from build123d import *

# Parameters (mm, degrees)
CROQUIS1_R              = 2.75
SALIENTE_EXTRUIR1_DEPTH = 6
SALIENTE_EXTRUIR2_DEPTH = 12
CORTAR_EXTRUIR1_DEPTH   = 4


with BuildPart() as part:
    # Croquis1 → Saliente-Extruir1 (new body)
    with BuildSketch(Plane.XY):
        Polygon((-9.5, 11.2), (-14, 11.2), (-14, 0), (0, 0), (0, 11.2), (-4.5, 11.2), (-4.5, 15.2), (-9.5, 15.2), align=None)
        with Locations((-7, 6)):
            Circle(CROQUIS1_R, mode=Mode.SUBTRACT)
    extrude(amount=SALIENTE_EXTRUIR1_DEPTH)

    # Croquis2 → Saliente-Extruir2 (add)
    with BuildSketch(Plane(origin=(0, 15.2, 0), x_dir=(1, 0, 0), z_dir=(0, 1, 0))):
        with BuildLine():
            Line((-9.5, 0), (-4.5, 0))
            ThreePointArc((-4.5, 0), (-7, -2.5), (-9.5, 0))
        make_face()
    extrude(amount=SALIENTE_EXTRUIR2_DEPTH)

    # Croquis3 → Cortar-Extruir1 (cut)
    with BuildSketch(Plane.XY.offset(6)):
        Polygon((-2.092522712, 6), (-4.546261356, 10.25), (-9.453738644, 10.25), (-11.907477288, 6), (-9.453738644, 1.75), (-4.546261356, 1.75), align=None)
    extrude(amount=-CORTAR_EXTRUIR1_DEPTH, mode=Mode.SUBTRACT)


solid = part.part
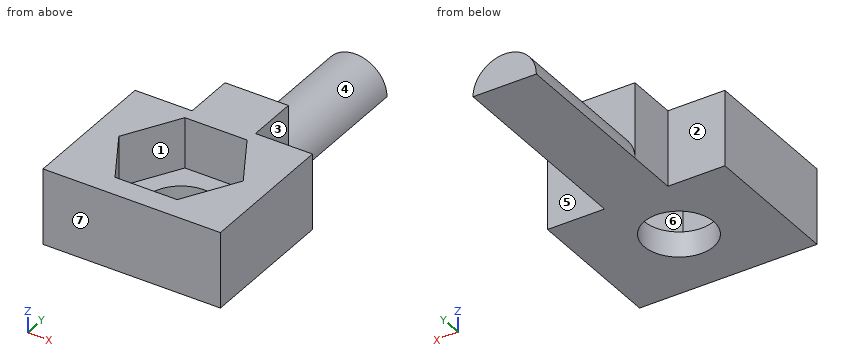
Can you work these out from the model? Positions are in its coordinate system, mm. Face numbers are marked on the shaded views. A direction names the side the tool comes from. Coordinates: 2 decimals unless noted, no trailing zeros. Write each loop counter-clockwise with the first axis right and the second up, starting at its lowest first coordinate (ties: lowest second). Pieces come first, ordered by that corner, then holes. Notation, with made-up numbers: M 44,76.5 L 58,76.5 A12 cw 58,97.5 Z; hole C 36.5,-7.75 d1. An arc over 180 degrees is marked long. Use one line per item in the form item = value.
Q1. I need wall thicknesses on line 1 along X through (y, z) = (6, 1.1); line 2 along Y through (x, z) = (-7, 1.05); line 3 along Y through (x, z) = (-4.75, 4). Which ranges of each line are inside material? Lowest first, please. Write a range as from..to.
Model answer:
line_1 = -14..-9.75, -4.25..0
line_2 = 0..3.25, 8.75..27.2
line_3 = 0..1.75, 10.25..15.2
Q2. If we section it at C-C (y = 4.5): Write out the boundary of the cut face in (x, z).
Model answer:
outline = M -14,0 L -9.3,0 L -9.3,2 L -11.04,2 L -11.04,6 L -14,6 Z; M -4.7,0 L 0,0 L 0,6 L -2.96,6 L -2.96,2 L -4.7,2 Z
Q3. For the marked faces 1, 2, 3 and 4, which set-ups out of +Z, -Z, +X, -X, +Y, -Y let a thin tool reach every point of the face, with its end or its side?
Model answer:
face_1 = +Z
face_2 = +Z, -Z, -X, +Y
face_3 = +Z, -Z, +X, +Y
face_4 = +Z, +Y
Q4. If we section it at A-A (x = -7): Write out the boundary of the cut face in (y, z), then the cut area to 3 significant figures.
Model answer:
outline = M 0,0 L 3.25,0 L 3.25,2 L 1.75,2 L 1.75,6 L 0,6 Z; M 8.75,0 L 27.2,0 L 27.2,2.5 L 15.2,2.5 L 15.2,6 L 10.25,6 L 10.25,2 L 8.75,2 Z
area = 76.2 mm^2
Q5. We'd pull the mould along Y, two halves only. Please class the marked faces 5, 6 and 7: +Y half, -Y half, draft (parallel to the pull), parting line (faces both ways), or undercut.
Model answer:
face_5 = +Y half
face_6 = undercut
face_7 = -Y half
Q6. If we section it at B-B (z = 4.85): Write out the boundary of the cut face in (x, y), then the cut area to 3 significant figures.
Model answer:
outline = M -14,0 L 0,0 L 0,11.2 L -4.5,11.2 L -4.5,15.2 L -9.5,15.2 L -9.5,11.2 L -14,11.2 Z; hole M -11.91,6 L -9.45,1.75 L -4.55,1.75 L -2.09,6 L -4.55,10.25 L -9.45,10.25 Z
area = 114 mm^2
Q7. For P1, Ø4, axis at x = -9, y = 6.5, coming from the +Z side; P2, Ø1.5, axis at x = -7, y = 6.5, coming from the -Z side; P3, Ø3.5, axis at x = -12, z = 2, coming from the +Y side; P4, Ø3, axis at x = -7.5, z = 4.5, coming from the -Y side, each with a flat end and sliding along its axis, tell me the tip position at first contact or that it passes through.
Model answer:
P1 = 2
P2 = through
P3 = 11.2
P4 = 0
Q8. If we section it at D-D (z = 1.5): Write out the boundary of the cut face in (x, y), then the cut area to 3 significant figures.
Model answer:
outline = M -14,0 L 0,0 L 0,11.2 L -4.5,11.2 L -4.5,15.2 L -5,15.2 L -5,27.2 L -9,27.2 L -9,15.2 L -9.5,15.2 L -9.5,11.2 L -14,11.2 Z; hole C -7,6 d5.5
area = 201 mm^2
